```python
from build123d import *

# Parameters (mm, degrees)
F1_DEPTH = 15.24
F2_SIZE  = 5.08


with BuildPart() as f1:
    # F0 (on Front) → F1 (new body)
    with BuildSketch(Plane.XZ):
        Polygon((0, 508), (0, 0), (25.4, 0), (50.8, 508), (175.280874, 729.405763), (172.053954, 762), (228.6, 762), (228.6, 812.8), (0, 812.8), (0, 762), (121.005602, 762), (124.269706, 729.030173), align=None)
    extrude(amount=F1_DEPTH)

    # F2
    f2_edges = [f1.edges().sort_by_distance(p)[0] for p in [
        (113.040437, -15.24, 618.702882),
        (38.1, -15.24, 254),
        (0, -15.24, 254),
        (62.134853, -15.24, 618.515087),
        (0, 0, 254),
        (62.134853, 0, 618.515087),
        (38.1, 0, 254),
        (113.040437, 0, 618.702882),
        (122.637654, 0, 745.515087),
        (173.667414, 0, 745.702882),
        (173.667414, -15.24, 745.702882),
        (122.637654, -15.24, 745.515087),
    ]]
    chamfer(f2_edges, length=F2_SIZE)


solid = f1.part
```
For this review, take the finished solid that the model builds, in its own axes (mm). A direction names the side the tool comes from. Coordinates: 2 decimals unless noted, no trailing zeros. Write each loop counter-clockwise with the first axis right and the second up, starting at its lowest first coordinate (ties: lowest second). Pieces come first, ordered by that corner, then holes.
(1) Wall thickness on probe 1 along Z at (x, y) = (87, -8); probe 2 along Z at (x, y) = (105.5, -1); probe 3 along Z at (x, y) = (197.5, -1): over which ranges is each line inside the solid? List them lowest first.
(2) Add section D-D on x = 35.5. Give the boundary of the cut face in (y, z).
(3) Add section C-C on y = -12.5. Give the boundary of the cut face in (x, z), then the cut area to 3 significant figures.
(4) For pin 1 Ø4.5 at (x, y) = (84.5, -4.5) entering from -Z; pin 2 Ø5 at (x, y) = (118, -3.5) entering from -Z; pin 3 Ø5 at (x, y) = (130, -9) entering from -Z, all flat-tipped, find the tip position at first contact; note any pin that passes through.
(5) The part is to be moulded in two halves that separate along Z. For faces 4 (the face through (109.627, -2.504, 617.887)), 5 (the face through (228.6, -8, 787)), 6 (the face through (63.005, -7.584, 620.062)), say which applies: +Z half, -Z half, draft (parallel to the pull), parting line (faces both ways), or undercut.
(6) Add section B-B on z = 170. Give the boundary of the cut face in (x, y), then the cut area to 3 significant figures.
(7) Tool access review of faces 1 (the face through (63, 0, 559)), 2 (the face through (65.6, -12.7, 619.5)), 3 (the face through (65.648, -2.504, 619.508)): name each direction out of +Z, -Z, +X, -X, +Y, -Y from which nothing blocks a thin tool from reaching the whole face with its end or side.
(8) Add section A-A on x = 112.5. Give the boundary of the cut face in (y, z), then the cut area to 3 significant figures.
Answer sheet:
1. probe 1: z = 572.39 to 662.74, 762 to 812.8
1. probe 2: z = 613.62 to 687.32, 762 to 812.8
1. probe 3: z = 762 to 812.8
2. outline: (-15.24, 303.73) - (-10.16, 202) - (-5.08, 202) - (0, 303.73) - (0, 560.78) - (-5.08, 571.14) - (-10.16, 571.14) - (-15.24, 560.78) - close; (-15.24, 762) - (0, 762) - (0, 812.8) - (-15.24, 812.8) - close
3. outline: (0, 762) - (123.36, 762) - (126.67, 728.53) - (2.34, 507.39) - (2.34, 0) - (23.06, 0) - (48.49, 508.67) - (172.88, 729.91) - (169.7, 762) - (228.6, 762) - (228.6, 812.8) - (0, 812.8) - close
3. area: 40,200 mm2
4. pin 1: stops at z = 564.07
4. pin 2: stops at z = 624.08
4. pin 3: stops at z = 644.42
5. face 4: -Z half
5. face 5: draft
5. face 6: undercut
6. outline: (0, -10.16) - (5.08, -15.24) - (28.81, -15.24) - (33.9, -10.16) - (33.9, -5.08) - (28.81, 0) - (5.08, 0) - (0, -5.08) - close
6. area: 465 mm2
7. face 1: +Z, -Z, +X, -X, +Y
7. face 2: -X, -Y
7. face 3: -X, +Y
8. outline: (-15.24, 628.11) - (-10.16, 617.74) - (-5.08, 617.74) - (0, 628.11) - (0, 697.73) - (-5.08, 708.1) - (-10.16, 708.1) - (-15.24, 697.73) - close; (-15.24, 762) - (0, 762) - (0, 812.8) - (-15.24, 812.8) - close
8. area: 2,050 mm2
